from build123d import *

# Parameters (mm, degrees)
BOSS_EXTRUDE1_DEPTH = 16
SHELL1_T            = 2.5
SKETCH2_W           = 12
SKETCH2_H           = 14
SKETCH2_H_2         = 5.195244662
CUT_EXTRUDE1_DEPTH  = 4
SKETCH3_W           = 2
SKETCH3_H           = 50
SKETCH3_W_2         = 1.814522713
BOSS_EXTRUDE2_DEPTH = 2
SKETCH4_W           = 31.017616101
SKETCH4_H           = 3.530460369
BOSS_EXTRUDE3_DEPTH = 2


with BuildPart() as part:
    # Sketch1 → Boss-Extrude1 (new body)
    with BuildSketch(Plane(origin=(0, 0, 0), x_dir=(1, 0, 0), z_dir=(0, 1, 0))):
        Polygon((0, 0), (0, 56), (7.260584432, 56), (13.399361706, 60.750217247), (49.399361706, 60.750217247), (56, 56), (58, 56), (58, 0), align=None)
    extrude(amount=BOSS_EXTRUDE1_DEPTH)

    # Shell1
    shell1_openings = [part.faces().sort_by_distance(p)[0] for p in [
        (29.147078279, 16, -29.765448683),
    ]]
    offset(amount=SHELL1_T, openings=shell1_openings, kind=Kind.INTERSECTION)

    # Sketch2 → Cut-Extrude1 (cut)
    with BuildSketch(Plane(origin=(0, 0, 0), x_dir=(-1, 0, 0), z_dir=(0, 0, -1))):
        with Locations((-47.5, 7)):
            Rectangle(SKETCH2_W, SKETCH2_H)
        with Locations((-30.5, 13.402377669)):
            Rectangle(SKETCH2_W, SKETCH2_H_2)
    extrude(amount=-CUT_EXTRUDE1_DEPTH, mode=Mode.SUBTRACT)

    # Sketch3 → Boss-Extrude2 (add)
    with BuildSketch(Plane(origin=(0, 0, 0), x_dir=(1, 0, 0), z_dir=(0, 1, 0))):
        with Locations((1, 27.58353092)):
            Rectangle(SKETCH3_W, SKETCH3_H)
        with Locations((56.968981121, 27.58353092)):
            Rectangle(SKETCH3_W_2, SKETCH3_H)
    extrude(amount=BOSS_EXTRUDE2_DEPTH)

    # Sketch4 → Boss-Extrude3 (add)
    with BuildSketch(Plane(origin=(0, 0, 0), x_dir=(1, 0, 0), z_dir=(0, 1, 0))):
        with Locations((31.80262956, 58.741489624)):
            Rectangle(SKETCH4_W, SKETCH4_H)
    extrude(amount=BOSS_EXTRUDE3_DEPTH)


solid = part.part
Geometry: final body of the model. Coordinates: model frame, mm. A direction names the side the tool comes from. Coordinates: 2 decimals unless noted, no trailing zeros. Write each loop counter-clockwise with the first axis right and the second up, starting at its lowest first coordinate (ties: lowest second). Pieces come first, ordered by that corner, then holes. Notation, with made-up numbers: (62.25, 6.5) - (88.25, 6.5) arc R23 ccw to (88.25, 14.5) - close; hole circle Ø11 at (-3.5, 30). An arc over 180 degrees is marked (long way). Return JSON: item names as keys, results as strings.
Item 1: Reachability of faces 5 (the face through (2, 7, -58.5)), 6 (the face through (53.5, 7, 1)), 7 (the face through (0, 8, -28)), 8 (the face through (24.5, 13, 1)), 9 (the face through (59, 16, -33)) from +Z, -Z, +X, -X, +Y, -Y: full face, straight path, thin tool, end or side. Return the list, or none.
Completed:
{"face 5": "-Z, -X, +Y, -Y", "face 6": "+Z", "face 7": "+Y", "face 8": "+Z, +Y", "face 9": "+Z, -Z, +X, -X, +Y"}
Item 2: Section query B-B (y = 11.75). Output: boundary loops of the cut face in (x, z).
Completed:
{"outline": "(-2.5, -58.5) - (6.41, -58.5) - (12.55, -63.25) - (50.21, -63.25) - (56.81, -58.5) - (60.5, -58.5) - (60.5, 2.5) - (53.5, 2.5) - (53.5, 0) - (58, 0) - (58, -56) - (56, -56) - (49.4, -60.75) - (13.4, -60.75) - (7.26, -56) - (0, -56) - (0, 0) - (24.5, 0) - (24.5, 2.5) - (-2.5, 2.5) - close; (36.5, 0) - (41.5, 0) - (41.5, 2.5) - (36.5, 2.5) - close"}
Item 3: Pin query (flat end, axial travel): pin 1 Ø1.5 at (x, z) = (57, -18.5) entering from +Y; pin 2 Ø1.1 at (x, y) = (58, 3) entering from -Z; pin 3 Ø10 at (x, y) = (3, 4) entering from -Z. Return the tip coordinate at first contact, or that it passes through.
Completed:
{"pin 1": "stops at y = 2", "pin 2": "stops at z = -58.5", "pin 3": "stops at z = -59.73"}
Item 4: Section query A-A (x = 44). Output: boundary loops of the cut face in (y, z), and give its area (3 significant figures).
Completed:
{"outline": "(-2.5, -63.25) - (16, -63.25) - (16, -60.75) - (0, -60.75) - (0, -60.51) - (2, -60.51) - (2, -56.98) - (0, -56.98) - (0, 2.5) - (-2.5, 2.5) - close; (14, 0) - (16, 0) - (16, 2.5) - (14, 2.5) - close", "area": "216 mm2"}
Item 5: Line query: L1, parallel to Z at x = 21, y = 1; L2, parallel to Z at x = 1.5, y = 10; L3, parallel to Z at x = 37, y = 12.5. Output: solid intervals per line, ascending.
Completed:
{"L1": "z = -63.25 to -60.75, -60.51 to -56.98, 0 to 2.5", "L2": "z = -58.5 to -56, 0 to 2.5", "L3": "z = -63.25 to -60.75, 0 to 2.5"}
Item 6: Pull-direction query (Z, two-part tool) for faces 1 (the face through (4, 8, -56)), 2 (the face through (53.46, 6.62, -60.91)), 3 (the face through (58, 8, -28)), 4 (the face through (47.311, 1, -59)); classes: +Z half, -Z half, draft (parallel to the pull), parting line (faces both ways), or undercut.
Completed:
{"face 1": "undercut", "face 2": "-Z half", "face 3": "undercut", "face 4": "draft"}
Item 7: Section query D-D (y = 7.5). Output: boundary loops of the cut face in (x, z), and give its area (3 significant figures).
Completed:
{"outline": "(-2.5, -58.5) - (6.41, -58.5) - (12.55, -63.25) - (50.21, -63.25) - (56.81, -58.5) - (60.5, -58.5) - (60.5, 2.5) - (53.5, 2.5) - (53.5, 0) - (58, 0) - (58, -56) - (56, -56) - (49.4, -60.75) - (13.4, -60.75) - (7.26, -56) - (0, -56) - (0, 0) - (41.5, 0) - (41.5, 2.5) - (-2.5, 2.5) - close", "area": "573 mm2"}
Item 8: Section query C-C (z = -30). Output: boundary loops of the cut face in (x, y), and give its area (3 significant figures).
Completed:
{"outline": "(-2.5, -2.5) - (60.5, -2.5) - (60.5, 16) - (58, 16) - (58, 0) - (57.88, 0) - (57.88, 2) - (56.06, 2) - (56.06, 0) - (2, 0) - (2, 2) - (0, 2) - (0, 16) - (-2.5, 16) - close", "area": "245 mm2"}
